Input: dimensioned drawing with shaded views. Units: mm. Origin: part minimum x, y, z. A direction names the side the tool comes from. Round coordinates to 2 decimals unless told otherwise and drop trailing zeros. Loops run counter-clockwise (first coordinate to the right, second up) from the corner with the lowest first, then second, coordinate; pieces in that order, holes last. Notation, with made-up numbers: (46, 59) -> (59, 59) arc R10 cw to (59, 65) -> close; hole circle Ø7 at (-31.5, 62). An arc over 180 degrees is marked (long way). Answer as a JSON object with one key per item and string values.
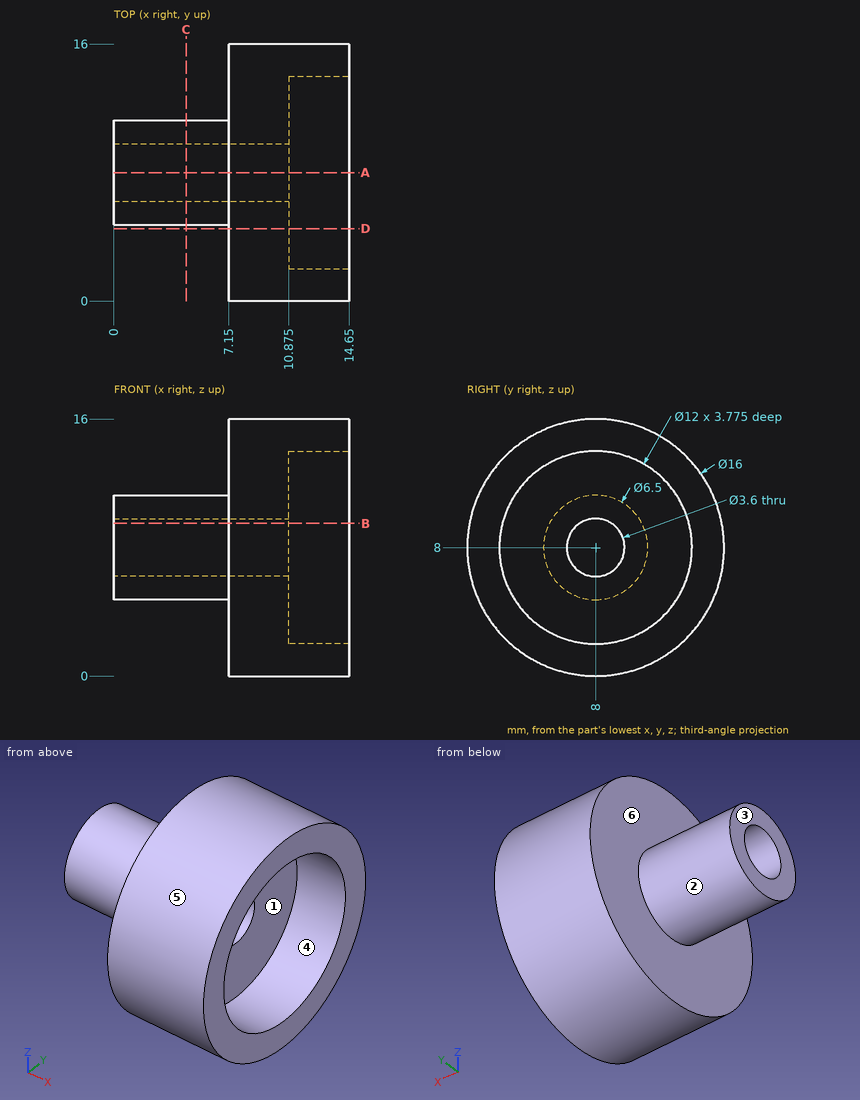
1) Draft query along Z for the marked faces 4, 5 and 6. Return one class per face: +Z half, -Z half, draft (parallel to the pull), parting line (faces both ways), or undercut.
Output:
{"face 4": "undercut", "face 5": "parting line", "face 6": "draft"}
2) Section D-D, the plane y = 4.5. Output: boundary loops of the cut face in (x, z) (3 decimals).
Output:
{"outline": "(7.15, 0.806) -> (14.65, 0.806) -> (14.65, 3.127) -> (10.875, 3.127) -> (10.875, 12.873) -> (14.65, 12.873) -> (14.65, 15.194) -> (7.15, 15.194) -> close"}
3) Contact query for flat-ended pins moving along their axis: P1, Ø2, axis at x = 11.5, z = 6.5, coming from the +Y side; P2, Ø8, axis at y = 5.5, z = 7, coming from the -X side; P3, Ø4, axis at x = 7.5, z = 12, coming from the +Y side; P4, Ø6, axis at x = 9.5, z = 12, coming from the +Y side. Output: stop coordinate, or through.
Output:
{"P1": "stops at y = 15.98", "P2": "stops at x = 0", "P3": "stops at y = 15.75", "P4": "stops at y = 15.94"}
4) Section B-B, the plane z = 9.5. Output: boundary loops of the cut face in (x, y) (3 decimals).
Output:
{"outline": "(0, 5.117) -> (7.15, 5.117) -> (7.15, 0.142) -> (14.65, 0.142) -> (14.65, 2.191) -> (10.875, 2.191) -> (10.875, 7.005) -> (0, 7.005) -> close; (0, 8.995) -> (10.875, 8.995) -> (10.875, 13.809) -> (14.65, 13.809) -> (14.65, 15.858) -> (7.15, 15.858) -> (7.15, 10.883) -> (0, 10.883) -> close"}
5) Section A-A, the plane y = 8. Output: boundary loops of the cut face in (x, z) (3 decimals), plus the area to 3 significant figures.
Output:
{"outline": "(0, 4.75) -> (7.15, 4.75) -> (7.15, 0) -> (14.65, 0) -> (14.65, 2) -> (10.875, 2) -> (10.875, 6.2) -> (0, 6.2) -> close; (0, 9.8) -> (10.875, 9.8) -> (10.875, 14) -> (14.65, 14) -> (14.65, 16) -> (7.15, 16) -> (7.15, 11.25) -> (0, 11.25) -> close", "area": "82.0 mm^2"}
6) Ray query, probe 1 along Y at (x, z) = (4, 8); probe 2 along Y at (x, z) = (7.75, 8); probe 3 along X at (y, z) = (11.5, 11.75) (3 decimals). Return the intervals inside material, ascending.
Output:
{"probe 1": "y = 4.75 to 6.2, 9.8 to 11.25", "probe 2": "y = 0 to 6.2, 9.8 to 16", "probe 3": "x = 7.15 to 10.875"}
7) Reachability of the marked faces 1, 2 and 3 from +Z, -Z, +X, -X, +Y, -Y: full face, straight path, thin tool, end or side. Return the list, or none.
Output:
{"face 1": "+X", "face 2": "-X", "face 3": "+Z, -Z, -X, +Y, -Y"}
8) Section C-C, the plane x = 4.5. Output: boundary loops of the cut face in (y, z), plus the area to 3 significant figures.
Output:
{"outline": "circle Ø6.5 at (8, 8); hole circle Ø3.6 at (8, 8)", "area": "23.0 mm^2"}
